Autodesk Fusion 360 part; units mm, degrees
sketch "Sketch1" plane through (0, 0, 0) normal (0, 1, 0) x (1, 0, 0)
  line L0 (0, 0) -> (65.7, 0)
  line L1 (65.7, 0) -> (65.7, 80.4)
  line L2 (65.7, 80.4) -> (0, 80.4)
  line L3 (0, 80.4) -> (0, 0)
  circle A0 centre (5, 5) radius 1.7
  circle A1 centre (60.7, 5) radius 1.7
  circle A2 centre (5, 75.4) radius 1.7
  line L4 (65.7, 80.4) -> (47.5, 80.4)
  line L5 (47.5, 80.4) -> (47.5, 73)
  line L6 (47.5, 73) -> (65.7, 73)
  line L7 (65.7, 73) -> (65.7, 80.4)
  line L8 (9.5, 78.4) -> (29.5, 78.4)
  line L9 (29.5, 78.4) -> (29.5, 74.9)
  line L10 (29.5, 74.9) -> (9.5, 74.9)
  line L11 (9.5, 74.9) -> (9.5, 78.4)
  line L12 (14.35, 26.7) -> (51.35, 26.7)
  line L13 (51.35, 26.7) -> (51.35, 18.7)
  line L14 (51.35, 18.7) -> (14.35, 18.7)
  line L15 (14.35, 18.7) -> (14.35, 26.7)
  line L16 (17.85, 68) -> (47.85, 68)
  line L17 (47.85, 68) -> (47.85, 48)
  line L18 (47.85, 48) -> (17.85, 48)
  line L19 (17.85, 48) -> (17.85, 68)
  circle A3 centre (21.91, 36.02) radius 6
  dimension "d1" = 65.7
  dimension "d2" = 80.4
  dimension "d3" = 3.4
  dimension "d4" = 5
  dimension "d5" = 5
  dimension "d7" = 3.4
  dimension "d8" = 5
  dimension "d9" = 5
  dimension "d11" = 3.4
  dimension "d12" = 5
  dimension "d13" = 5
  dimension "d15" = 18.2
  dimension "d16" = 7.4
  dimension "d17" = 20
  dimension "d18" = 3.5
  dimension "d19" = 2
  dimension "d20" = 9.5
  dimension "d27" = 37
  dimension "d28" = 8
  dimension "d30" = 30
  dimension "d31" = 20
  dimension "d34" = 12
  dimension "d36" = 9.32
  dimension "d43" = 17.85
extrude "Extrude1" add sketch "Sketch1" along normal blind 3 contours L0 L1 L2 L3 L5 L6
fillet "Fillet1" radius 5 3 edges at (65.7, 1.5, 0) (0, 1.5, 0) (0, 1.5, -80.4)
fillet "Fillet2" radius 1 8 edges at (17.85, 1.5, -68) (14.35, 1.5, -26.7) (47.85, 1.5, -68) (51.35, 1.5, -26.7) (51.35, 1.5, -18.7) (47.85, 1.5, -48) (17.85, 1.5, -48) (14.35, 1.5, -18.7)
For this review, take the finished solid that the model builds, in its own axes (mm). A direction names the side the tool comes from. Give positions to 0.01 mm unless a question says otherwise; leave off trailing zeros. Loops run counter-clockwise (first coordinate to the right, second up) from the corner with the lowest first, then second, coordinate; pieces in that order, holes last. Notation, with made-up numbers: M -10,88.25 L 7,88.25 A19 cw 7,104.25 Z; hole C -33.75,78 d7. An arc over 180 degrees is marked long. Put each result on its own line as item: value. Start each with the question number.
(1) Machinability: for faces 5 (the flat face through (32, 0, -32)), 6 (the flat face through (47.5, 1, -77)), 7 (the flat face through (14.35, 1, -23)), which of the approach directions +Z, -Z, +X, -X, +Y, -Y give a long, thin tool a straight path to every point of the face, cutting with its end or side? Answer none if there is none.
(2) Add section B-B, the plane x = 21.91. Write out the cut boundary in (y, z).
(3) Add section C-C, the plane y = 1.4. Give the number of separate pieces and of enclosed holes in the cut face, then the cut area to 3 significant figures.
(4) The part is to be moulded in two halves that separate along Z. For faces 1 (the flat face through (27, 1, -80.4)), 2 (the cylindrical face through (59.35, 1.48, -6.03)), 3 (the flat face through (33, 1, -18.7)), 4 (the cylindrical face through (1, 2, -2)), say which applies: +Z half, -Z half, draft (parallel to the pull), parting line (faces both ways), or undercut.
(5) For pin 1 (1.5 mm diameter, centred on y = 2, z = -77, fed in from -X); pin 2 (0.9 mm diameter, centred on x = 60, y = 1, fed in from -Z); pin 3 (0.9 mm diameter, centred on y = 1.5, z = -76, fed in from +X); pin 4 (2.5 mm diameter, centred on x = 5, z = -75.4, fed in from +Y), all flat-tipped, find the tip position at first contact; note any pin that passes through.
(6) Add section A-A, the plane z = -36.02. Write out the cut boundary in (x, y), then the cut area to 3 significant figures.
(7) Wall thickness on L1, parallel to Z at x = 44.5, y = 1.5; L2, parallel to X at y = 2.2, z = -5; L3, parallel to Z at x = 5, y = 1.9: over which ranges is each line inside the solid? List them lowest first.
(8) Add section D-D, the plane x = 41.5. Write out the cut boundary in (y, z), then the cut area to 3 significant figures.
Result:
1. face 5: +Z, -Z, +X, -X, -Y
1. face 6: -Z, +X, +Y, -Y
1. face 7: +Y, -Y
2. outline: M 0,-80.4 L 3,-80.4 L 3,-78.4 L 0,-78.4 Z; M 0,-74.9 L 3,-74.9 L 3,-68 L 0,-68 Z; M 0,-48 L 3,-48 L 3,-42.02 L 0,-42.02 Z; M 0,-30.02 L 3,-30.02 L 3,-26.7 L 0,-26.7 Z; M 0,-18.7 L 3,-18.7 L 3,0 L 0,0 Z
3. separate pieces: 1
3. enclosed holes: 7
3. area: 4,030 mm^2
4. face 1: -Z half
4. face 2: undercut
4. face 3: undercut
4. face 4: +Z half
5. pin 1: stops at x = 0.07
5. pin 2: stops at z = -73
5. pin 3: stops at x = 47.5
5. pin 4: passes through
6. outline: M 0,0 L 15.91,0 L 15.91,3 L 0,3 Z; M 27.91,0 L 65.7,0 L 65.7,3 L 27.91,3 Z
6. area: 161 mm^2
7. L1: z = -80.4 to -68, -48 to -26.7, -18.7 to 0
7. L2: x = 0 to 3.3, 6.7 to 59, 62.4 to 65.7
7. L3: z = -80.4 to -77.1, -73.7 to -6.7, -3.3 to 0
8. outline: M 0,-80.4 L 3,-80.4 L 3,-68 L 0,-68 Z; M 0,-48 L 3,-48 L 3,-26.7 L 0,-26.7 Z; M 0,-18.7 L 3,-18.7 L 3,0 L 0,0 Z
8. area: 157 mm^2
